from build123d import *

# Parameters (mm, degrees)
BOSS_EXTRUDE1_START = -59
SKETCH1_R           = 5
BOSS_EXTRUDE1_DEPTH = 6


with BuildPart() as part:
    # Sketch1 → Boss-Extrude1 (new body)
    with BuildSketch(Plane.XY.offset(BOSS_EXTRUDE1_START)):
        with BuildLine():
            Line((-253.286796564, -275.955844123), (-275.955844123, -253.286796564))
            ThreePointArc((-275.955844123, -253.286796564), (-289.033326685, -250.685523549), (-296.441125497, -261.772077939))
            Line((-296.441125497, -261.772077939), (-296.441125497, -284.441125497))
            ThreePointArc((-296.441125497, -284.441125497), (-292.926406871, -292.926406871), (-284.441125497, -296.441125497))
            Line((-284.441125497, -296.441125497), (-261.772077939, -296.441125497))
            ThreePointArc((-261.772077939, -296.441125497), (-250.685523549, -289.033326685), (-253.286796564, -275.955844123))
        make_face()
        with Locations((-278.763455967, -278.763455967)):
            Circle(SKETCH1_R, mode=Mode.SUBTRACT)
    extrude(amount=BOSS_EXTRUDE1_DEPTH)


solid = part.part
Design review of the part built by this model. Coordinates are the model's own, in mm. Coordinates: 2 decimals unless noted, no trailing zeros. Loops run counter-clockwise (first coordinate to the right, second up) from the corner with the lowest first, then second, coordinate; pieces in that order, holes last. Notation, with made-up numbers: (-10.75, -5.5) - (15.25, -5.5) arc R20 cw to (15.25, 9.5) - close; hole circle Ø10 at (1, -14.75). An arc over 180 degrees is marked (long way). Use CSV: the item, a comma, the result in double quotes. Start each with the question number.
1. Add section B-B on z = -54.3. Give the boundary of the cut face in (x, y).
2. Add section C-C on y = -259.5. Give the boundary of the cut face in (x, z).
3. Clearance check with flat-ended pins moving along their axes: pin 1 (8 mm diameter, centred on x = -278.76, y = -278.76, fed in from -Z) (1 decimal); pin 2 (1.5 mm diameter, centred on x = -278.5, z = -57.5, fed in from +Y). State where each tip first meets the part, or that it passes through.
4. Add section A-A on x = -281. Give the boundary of the cut face in (y, z).
5. Add section D-D on x = -275. Give the boundary of the cut face in (y, z).
6. To check wall thickness, follow probe 1 along Y at (x, z) = (-283, -55.35); probe 2 along X at (y, z) = (-281.5, -56.3); probe 3 along X at (y, z) = (-281, -57.45). State the ranges of each line that lie inside material, in increasing order.
7. Mouldability with a two-part tool opening along X and no side actions: class faces 1 (the flat face through (-273, -296.441, -56)), 2 (the flat face through (-264.46, -264.78, -56.04)), 3 (the cylindrical face through (-276.075, -274.547, -56.042)) as released by +X, released by -X, zero draft, split by the parting line, or undercut.
Resolved:
1,outline,"(-296.44, -284.44) arc R12 ccw to (-284.44, -296.44) - (-261.77, -296.44) arc R12 ccw to (-253.29, -275.96) - (-275.96, -253.29) arc R12 ccw to (-296.44, -261.77) - close; hole circle Ø10 at (-278.76, -278.76)"
2,outline,"(-296.22, -59) - (-269.74, -59) - (-269.74, -53) - (-296.22, -53) - close"
3,pin 1,"through"
3,pin 2,"y = -250.95"
4,outline,"(-296.44, -59) - (-283.24, -59) - (-283.24, -53) - (-296.44, -53) - close; (-274.29, -59) - (-250.28, -59) - (-250.28, -53) - (-274.29, -53) - close"
5,outline,"(-296.44, -59) - (-282.06, -59) - (-282.06, -53) - (-296.44, -53) - close; (-275.47, -59) - (-254.24, -59) - (-254.24, -53) - (-275.47, -53) - close"
6,probe 1,"-296.44 to -281.42, -276.11 to -249.86"
6,probe 2,"-296.44 to -282.95, -274.58 to -250.14"
6,probe 3,"-296.44 to -283.24, -274.29 to -250.28"
7,face 1,"zero draft"
7,face 2,"released by +X"
7,face 3,"undercut"
